Work out the finished part from the listing and answer in its coordinate system (mm). Coordinates: 2 decimals unless noted, no trailing zeros. Write each loop counter-clockwise with the first axis right and the second up, starting at its lowest first coordinate (ties: lowest second). Pieces come first, ordered by that corner, then holes. Notation, with made-up numbers: (-21.75, -1.75) -> (36.25, -1.75) arc R12 cw to (36.25, 21.25) -> close; hole circle Ø9 at (-33, -31.75). An arc over 180 degrees is marked (long way). Write each question's results on one line, items separated by ' | '. Start each with the question number.
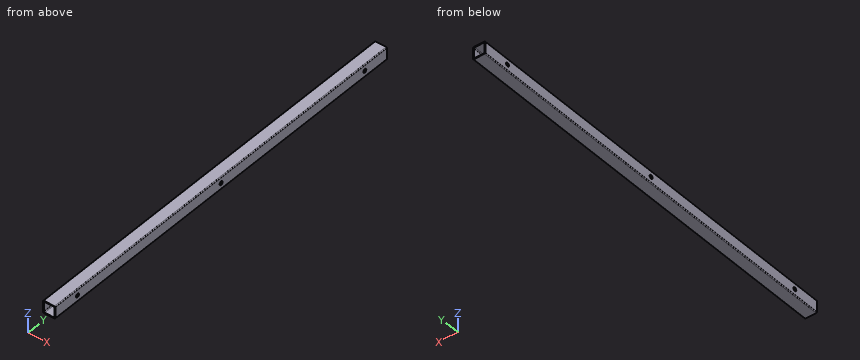
from build123d import *

# Parameters (mm, degrees)
SKETCH1_W                  = 19.304
SKETCH1_H                  = 19.304
SKETCH1_W_2                = 16.764
SKETCH1_H_2                = 16.764
BOSS_EXTRUDE1_DEPTH        = 645.16
FILLET1_R                  = 1.27
F_1_0_228_DIAMETER_HOLE1_D = 5.7912


with BuildPart() as part:
    # Sketch1 → Boss-Extrude1 (new body)
    with BuildSketch(Plane(origin=(0, 0, 0), x_dir=(1, 0, 0), z_dir=(0, 1, 0))):
        Rectangle(SKETCH1_W, SKETCH1_H)
        Rectangle(SKETCH1_W_2, SKETCH1_H_2, mode=Mode.SUBTRACT)
    extrude(amount=BOSS_EXTRUDE1_DEPTH)

    # Fillet1
    fillet1_edges = [part.edges().sort_by_distance(p)[0] for p in [
        (-8.382, 322.58, 8.382),
        (8.382, 322.58, 8.382),
        (8.382, 322.58, -8.382),
        (-8.382, 322.58, -8.382),
        (9.652, 322.58, 9.652),
        (-9.652, 322.58, 9.652),
        (-9.652, 322.58, -9.652),
        (9.652, 322.58, -9.652),
    ]]
    fillet(fillet1_edges, radius=FILLET1_R)

    # #1 (0.228) Diameter Hole1 (through all)
    with Locations(Plane(origin=(9.652, 0, 0), x_dir=(0, 0, -1), z_dir=(1, 0, 0))):
        with Locations((0, 43.18), (0, 601.98), (0, 322.58)):
            Hole(F_1_0_228_DIAMETER_HOLE1_D / 2)


solid = part.part
1. Find section A-A on y = 483. Give the vertices of the cut face in (x, z), and give its area (3 significant figures).
2. Find section B-B on x = 2.5. Give the vertices of the cut face in (y, z).
3. Find the intervals of material crossed by L1, parallel to Y at x = 9.15, z = 0; L2, parallel to Z at x = 4, y = 162.5, in increasing order.
4. Find section C-C on z = 0. Give the number of separate pieces and of enclosed holes in the cut face, and give its area (3 significant figures).
Ans:
1) outline: (-9.65, -8.38) arc R1.27 ccw to (-8.38, -9.65) -> (8.38, -9.65) arc R1.27 ccw to (9.65, -8.38) -> (9.65, 8.38) arc R1.27 ccw to (8.38, 9.65) -> (-8.38, 9.65) arc R1.27 ccw to (-9.65, 8.38) -> close; hole (-8.38, -7.11) arc R1.27 ccw to (-7.11, -8.38) -> (7.11, -8.38) arc R1.27 ccw to (8.38, -7.11) -> (8.38, 7.11) arc R1.27 ccw to (7.11, 8.38) -> (-7.11, 8.38) arc R1.27 ccw to (-8.38, 7.11) -> close | area: 91.6 mm²
2) outline: (0, -9.65) -> (645.16, -9.65) -> (645.16, -8.38) -> (0, -8.38) -> close; (0, 8.38) -> (645.16, 8.38) -> (645.16, 9.65) -> (0, 9.65) -> close
3) L1: y = 0 to 40.28, 46.08 to 319.68, 325.48 to 599.08, 604.88 to 645.16 | L2: z = -9.65 to -8.38, 8.38 to 9.65
4) separate pieces: 8 | enclosed holes: 0 | area: 1,590 mm²
